Input: part model. Units: mm. Frame: model coordinates. Face numbers are marked on the shaded views. A direction names the side the tool comes from. Coordinates: 2 decimals unless noted, no trailing zeros. Write each loop counter-clockwise with the first axis right and the second up, starting at its lowest first coordinate (ties: lowest second). Pieces come first, ordered by that corner, then holes. Notation, with made-up numbers: (-10.75, -14) -> (26.25, -14) arc R29 ccw to (26.25, 8) -> close; hole circle Ø5 at (5.25, -9.5). An arc over 180 degrees is marked (long way). Use one line per item in the form item = value. Start each with the question number.
(1) Pull-direction query (X, two-part tool) for the marked faces 4, 5, 6 and 7; classes: released by +X, released by -X, zero draft, split by the parting line, or undercut.
(2) Ray query, line 1 along Z through (x, y) = (10, 5); line 2 along Z through (x, y) = (0.5, 35); line 3 along X through (y, z) = (8.5, 29.5). Return the intervals inside material, ascending.
(3) Cut plane B-B on z = -27.5. Return the cut outline in (x, y), plus the area to 3 significant figures.
(4) Cut plane A-A on x = 0. Return the cut outline in (y, z), plus the area to 3 significant figures.
(5) Set-up query: the marked faces 1, 2 and 3. Return all of +Z, -Z, +X, -X, +Y, -Y with unobstructed straight access to the full face (end or side cutting, diameter ignored); none if empty.
(6) First-contact query: pin 1 (12 mm diameter, centred on x = 2, z = -26, fed in from +Y); pin 2 (1.1 mm diameter, centred on y = 9.5, z = -43.5, fed in from -X); pin 3 (4 mm diameter, centred on x = 26.5, y = 25, fed in from -Z); pin 4 (5 mm diameter, centred on y = 17, z = -34.5, fed in from -X). Flat tips, straight axial feed; report the tip coordinate or a pass-through.
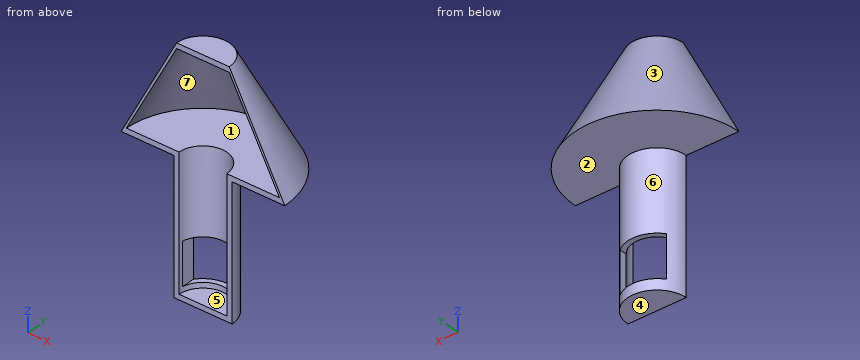
```python
from build123d import *

# Parameters (mm, degrees)
F1_ANGLE = 180
F2_W     = 20
F2_H     = 20
F3_DEPTH = 25


with BuildPart() as f1:
    # F0 (on Right) → F1 (revolve, symmetric)
    with BuildSketch(Plane.YZ) as f1_sk:
        Polygon((0, -60), (0, -62.5), (13.814939, -62.5), (13.814939, 0), (38.814939, 0), (12.5, 50), (0, 50), (0, 47.5), (12.5, 47.5), (36.314939, 2.5), (11.314939, 2.5), (11.314939, -60), align=None)
    revolve(axis=Axis((0, 0, -61.25), (0, 0, 1)), revolution_arc=F1_ANGLE / 2)
    revolve(f1_sk.sketch, axis=Axis((0, 0, -61.25), (0, 0, -1)), revolution_arc=F1_ANGLE / 2)

    # F2 (on Front) → F3 (cut)
    with BuildSketch(Plane.XZ):
        with Locations((-1.185061, -47.5)):
            Rectangle(F2_W, F2_H)
    extrude(amount=-F3_DEPTH, mode=Mode.SUBTRACT)


solid = f1.part
```
Values:
q1.face_4 = zero draft
q1.face_5 = undercut
q1.face_6 = split by the parting line
q1.face_7 = undercut
q2.line_1 = -62.5 to -60, 47.5 to 50
q2.line_2 = 0 to 2.5, 4.98 to 7.24
q2.line_3 = -21.68 to -20.32, 20.32 to 21.68
q3.outline = (-13.81, 0) -> (-11.31, 0) arc R11.31 cw to (11.31, 0) -> (13.81, 0) arc R13.81 ccw to start
q3.area = 98.7 mm2
q4.outline = (0, -62.5) -> (13.81, -62.5) -> (13.81, -57.5) -> (11.31, -57.5) -> (11.31, -60) -> (0, -60) -> close; (0, 47.5) -> (12.5, 47.5) -> (36.31, 2.5) -> (11.31, 2.5) -> (11.31, -37.5) -> (13.81, -37.5) -> (13.81, 0) -> (38.81, 0) -> (12.5, 50) -> (0, 50) -> close
q4.area = 291 mm2
q5.face_1 = -Y
q5.face_2 = -Z, +Y
q5.face_3 = +Z, +Y
q6.pin_1 = 13.81
q6.pin_2 = 8.81
q6.pin_3 = 0
q6.pin_4 = through
